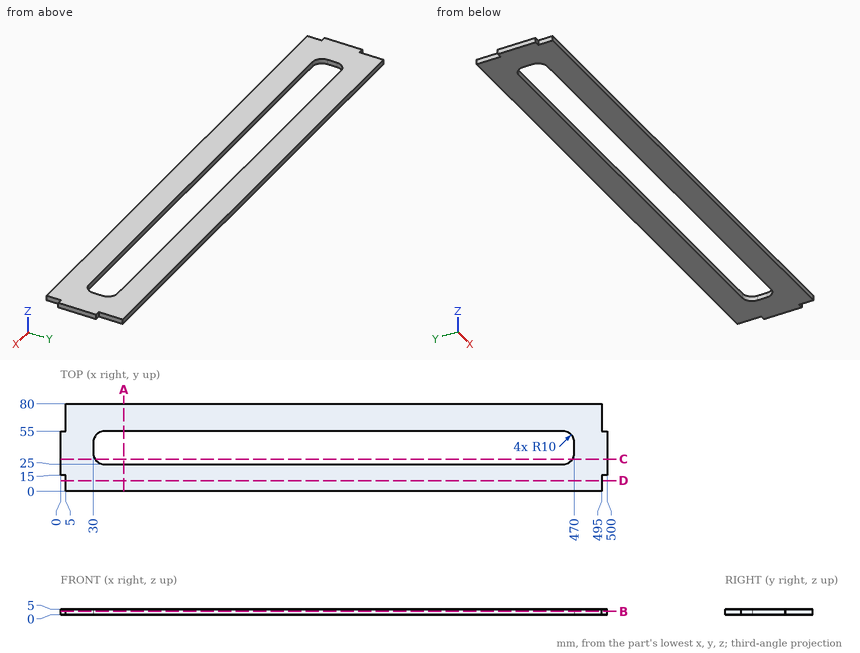
Job drawing, mm, ordinate dimensions from the low corner. One solid piece. Coordinates: 2 decimals unless noted, no trailing zeros. Write each loop counter-clockwise with the first axis right and the second up, starting at its lowest first coordinate (ties: lowest second). Pieces come first, ordered by that corner, then holes. Notation, with made-up numbers: (79, -1) - (127, -1) arc R9 ccw to (127, 3) - close; hole circle Ø9 at (-11.5, 52.5). An arc over 180 degrees is marked (long way). Use a Markdown table: item, result. Add a question column.
Item 1: Band-saw the part on D-D, the plane y = 10. Give the cut face in (x, z).
Item 2: Flat gauge pins, fed straight in: pin 1 (2 mm diameter, centred on y = 70.5, z = 2.5, fed in from +X); pin 2 (2.5 mm diameter, centred on x = 347, z = 3.5, fed in from -Y); pin 3 (2.5 mm diameter, centred on y = 64.5, z = 2.5, fed in from -X); pin 4 (1.5 mm diameter, centred on x = 497.5, z = 2, fed in from -Y). Where does each tip first touch, or does it go through?
Item 3: Band-saw the part on B-B, the plane z = 3.25. Give the cut face in (x, y), and give its area (3 significant figures).
Item 4: Band-saw the part on A-A, the plane x = 58. Give the cut face in (y, z), and give its area (3 significant figures).
Item 5: Drill centre lines: L1, parallel to Y at x = 337, z = 3.9; L2, parallel to X at y = 10, z = 0.4; L3, parallel to X at y = 38.5, z = 4. Where is each one in solid material? Low to high. Write a range as from..to.
Item 6: Band-saw the part on C-C, the plane y = 29.5. Give the cut face in (x, z), and give its area (3 significant figures).
Numbers:
| question | item | result |
|---|---|---|
| 1 | outline | (5, 0) - (495, 0) - (495, 5) - (5, 5) - close |
| 2 | pin 1 | x = 495 |
| 2 | pin 2 | y = 0 |
| 2 | pin 3 | x = 5 |
| 2 | pin 4 | y = 15 |
| 3 | outline | (0, 15) - (5, 15) - (5, 0) - (495, 0) - (495, 15) - (500, 15) - (500, 55) - (495, 55) - (495, 80) - (5, 80) - (5, 55) - (0, 55) - close; hole (30, 35) arc R10 ccw to (40, 25) - (460, 25) arc R10 ccw to (470, 35) - (470, 45) arc R10 ccw to (460, 55) - (40, 55) arc R10 ccw to (30, 45) - close |
| 3 | area | 26,500 mm2 |
| 4 | outline | (0, 0) - (25, 0) - (25, 5) - (0, 5) - close; (55, 0) - (80, 0) - (80, 5) - (55, 5) - close |
| 4 | area | 250 mm2 |
| 5 | L1 | 0..25, 55..80 |
| 5 | L2 | 5..495 |
| 5 | L3 | 0..30, 470..500 |
| 6 | outline | (0, 0) - (31.65, 0) - (31.65, 5) - (0, 5) - close; (468.35, 0) - (500, 0) - (500, 5) - (468.35, 5) - close |
| 6 | area | 316 mm2 |
